The model under review builds one solid part; all positions refer to its coordinate system, in mm. A direction names the side the tool comes from. Coordinates: 2 decimals unless noted, no trailing zeros. Order: outer loops, then holes, each group sorted by start corner. A loop starts at its lowest first (then second) coordinate and runs counter-clockwise, first axis right, second up. Notation, with made-up numbers: (-14.5, -38.75) -> (-2.5, -38.75) arc R30 cw to (-2.5, -6.75) -> close; hole circle Ø10 at (80, 5.5). An arc over 180 degrees is marked (long way). Put each result on its own line as item: value.
from build123d import *

# Parameters (mm, degrees)
F0_W     = 304.8
F0_H     = 457.2
F2_DEPTH = 25.4
F3_T     = -6.35
F4_W     = 3.175
F4_H     = 25.4


# Not quite as in the source:
# - the program builds the solid bodies; features that only make, move or delete a surface that nothing else refers to are left out


with BuildPart() as f2:
    # F0 (on Front) → F2 (new body)
    with BuildSketch(Plane.XZ):
        with Locations((152.4, -228.6)):
            Rectangle(F0_W, F0_H)
    extrude(amount=F2_DEPTH)

    # F3
    f3_openings = [f2.faces().sort_by_distance(p)[0] for p in [
        (152.4, 0, -228.6),
    ]]
    offset(amount=F3_T, openings=f3_openings)

    # F4 (on Right) → F5 (revolve)
    with BuildSketch(Plane.YZ):
        with Locations((1.5875, -12.7)):
            Rectangle(F4_W, F4_H)
    revolve(axis=Axis((0, 0, 39.7453531623), (0, 0, 1)))


solid = f2.part
Item 1: For pin 1 Ø6 at (y, z) = (-16.5, -258) entering from -X; pin 2 Ø6 at (x, z) = (214, -312.5) entering from +Y, all flat-tipped, find the tip position at first contact; note any pin that passes through.
Answers below:
pin 1: x = 0
pin 2: y = -19.05
Item 2: Consider section C-C on x = 227. Write out the cut boundary in (y, z).
Answers below:
outline: (-25.4, -457.2) -> (0, -457.2) -> (0, -450.85) -> (-19.05, -450.85) -> (-19.05, -6.35) -> (0, -6.35) -> (0, 0) -> (-25.4, 0) -> close
Item 3: For line 1 (X direction, y = -19, z = -312.5); line 2 (Z direction, x = 212.5, y = -17.5); line 3 (Y direction, x = 214.5, z = -271.5), list the stretches that pass through material, from the lowest coordinate up. Write a range as from..to.
Answers below:
line 1: 0..6.35, 298.45..304.8
line 2: -457.2..-450.85, -6.35..0
line 3: -25.4..-19.05
Item 4: Consider section A-A on y = -8.75. Write out the cut boundary in (x, z).
Answers below:
outline: (0, -457.2) -> (304.8, -457.2) -> (304.8, 0) -> (0, 0) -> close; hole (6.35, -450.85) -> (298.45, -450.85) -> (298.45, -6.35) -> (6.35, -6.35) -> close
Item 5: Mouldability with a two-part tool opening along X and no side actions: class faces 3 (the flat face through (150, -13, -457.2)), 4 (the flat face through (150, -9, -6.35)), 5 (the flat face through (304.8, -13, -232)) as +X half, -X half, draft (parallel to the pull), parting line (faces both ways), or undercut.
Answers below:
face 3: draft
face 4: undercut
face 5: +X half
Item 6: Consider section B-B on z = -70.5. Write out the cut boundary in (x, y).
Answers below:
outline: (0, -25.4) -> (304.8, -25.4) -> (304.8, 0) -> (298.45, 0) -> (298.45, -19.05) -> (6.35, -19.05) -> (6.35, 0) -> (0, 0) -> close
Item 7: For faces 1 (the flat face through (6.35, -9, -232)), 2 (the flat face through (150, -25.4, -225)), list the 3-axis set-ups (+Z, -Z, +X, -X, +Y, -Y) from which the entire face can be reached by the end or side of a thin tool; tool diameter is ignored.
Answers below:
face 1: +Y
face 2: +Z, -Z, +X, -X, -Y
